Could you check a few things on this model? Use its own coordinates, in mm. Face numbers are marked on the shaded views. A direction names the side the tool comes from. Round coordinates to 2 decimals unless told otherwise and drop trailing zeros. Write each loop counter-clockwise with the first axis right and the second up, starting at its lowest first coordinate (ties: lowest second). Pieces come first, ordered by that corner, then holes. Notation, with made-up numbers: (15, -28.75) -> (19, -28.75) arc R7 cw to (19, -15.75) -> close; hole circle Ø8 at (85.5, 4). An arc over 180 degrees is marked (long way). Return JSON: item names as keys, results as strings.
from build123d import *

# Parameters (mm, degrees)
F0_W     = 290.5125
F0_H     = 290.5125
F1_DEPTH = 1.5875
F2_W     = 293.6875
F2_H     = 293.6875
F2_W_2   = 290.5125
F2_H_2   = 290.5125
F3_DEPTH = 69.85


# Not quite as in the source:
# - a length typed as a fraction of an inch, garbled in the dataset ("3 / 203.2 mm" for 3/8 in), is restored


with BuildPart() as f1:
    # F0 (on Top) → F1 (new body)
    with BuildSketch(Plane.XY):
        with Locations((145.25625, 145.25625)):
            Rectangle(F0_W, F0_H)
    extrude(amount=F1_DEPTH)

    # F2 (on face) → F3 (join)
    with BuildSketch(Plane(origin=(0, 0, 0), x_dir=(1, 0, 0), z_dir=(0, 0, -1))):
        with Locations((145.25625, -145.25625)):
            Rectangle(F2_W, F2_H)
        with Locations((145.25625, -145.25625)):
            Rectangle(F2_W_2, F2_H_2, mode=Mode.SUBTRACT)
    extrude(amount=-F3_DEPTH)


solid = f1.part
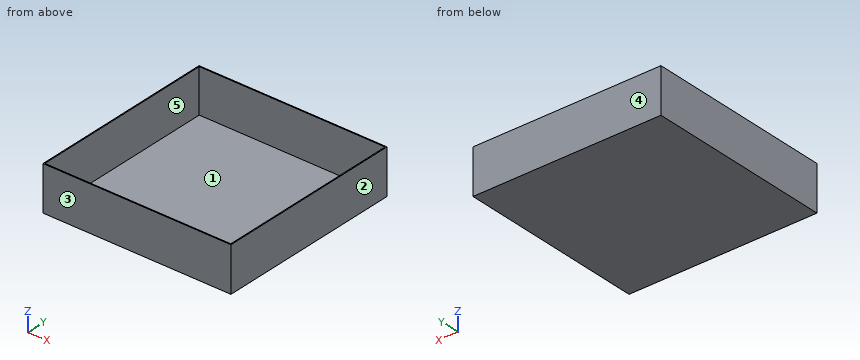
1) Thinking about a two-plate mould opening in X: for the marked faces 1, 2 and 3, which applies, pulls with the +X half, pulls with the -X half, needs draft (parallel to the pull), parting line crosses it, or undercut?
Return value:
{"face 1": "undercut", "face 2": "pulls with the +X half", "face 3": "needs draft"}
2) If I drill on probe 1 along X at (y, z) = (254, 62); probe 2 along Z at (x, y) = (243, 38), over which ranges is the centre line in solid material (lowest first)? Write a range as [from, to].
Return value:
{"probe 1": "[-1.59, 0], [290.51, 292.1]", "probe 2": "[0, 1.59]"}
3) I want a section at A-A, the plane z = 41.5. Please give me the cut outline in (x, y).
Return value:
{"outline": "(-1.59, -1.59) -> (292.1, -1.59) -> (292.1, 292.1) -> (-1.59, 292.1) -> close; hole (0, 0) -> (290.51, 0) -> (290.51, 290.51) -> (0, 290.51) -> close"}
4) Will this pin go through, and if not, where does the flat tip stop? pin 1 Ø2 at (x, y) = (166, 69) entering from +Z.
Return value:
{"pin 1": "z = 1.59"}
5) For the marked faces 4 and 5, which set-ups out of +Z, -Z, +X, -X, +Y, -Y let a thin tool reach every point of the face, with its end or its side?
Return value:
{"face 4": "+Z, -Z, +X, -X, +Y", "face 5": "+Z"}
6) I want a section at B-B, the plane y = 68.5. Please give me the cut outline in (x, z).
Return value:
{"outline": "(-1.59, 0) -> (292.1, 0) -> (292.1, 69.85) -> (290.51, 69.85) -> (290.51, 1.59) -> (0, 1.59) -> (0, 69.85) -> (-1.59, 69.85) -> close"}
